Verification items for this drawing (mm, ordinates from the low corner). Give positions to 0.01 mm unless a question says otherwise; leave off trailing zeros. Loops run counter-clockwise (first coordinate to the right, second up) from the corner with the lowest first, then second, coordinate; pieces in that order, holes last. Notation, with made-up numbers: (-16.75, 1) -> (-5.75, 1) arc R27 cw to (-5.75, 30) -> close; hole circle Ø4 at (22.25, -7). An arc over 180 degrees is marked (long way). Answer as a JSON object with one key per item and string values.
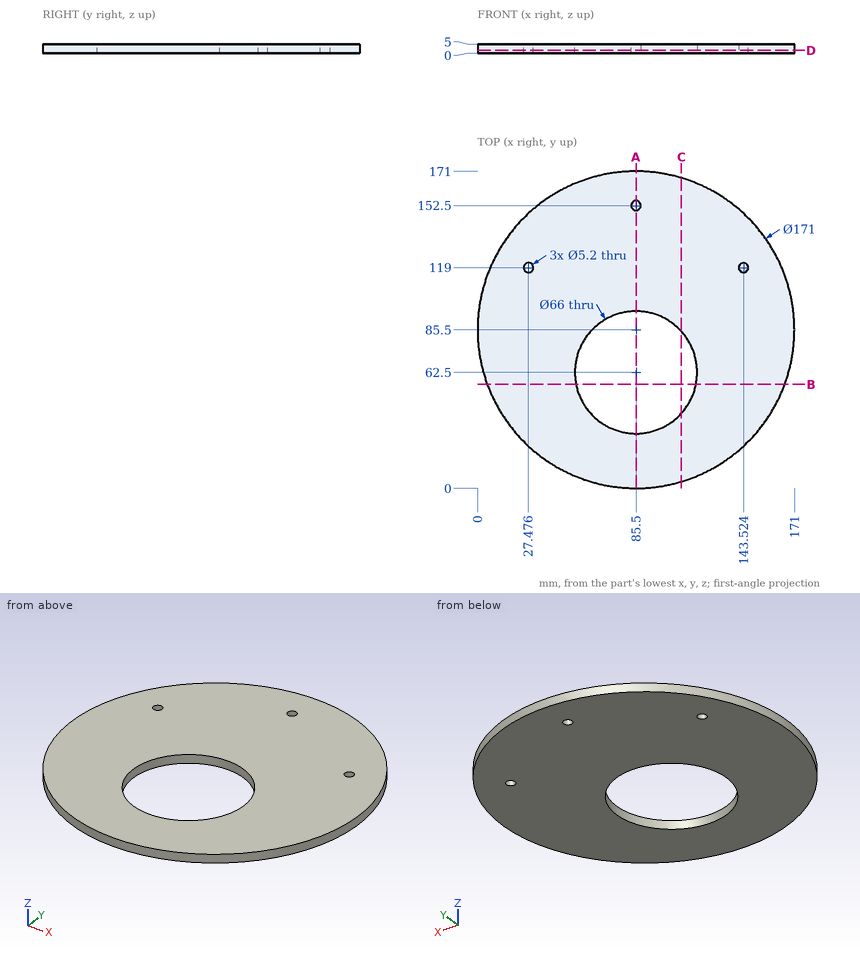
1) Section check B-B on y = 56. Record the cut outline in (x, z), plus the area to 3 significant figures.
Geometry check:
{"outline": "(5.25, 0) -> (53.15, 0) -> (53.15, 5) -> (5.25, 5) -> close; (117.85, 0) -> (165.75, 0) -> (165.75, 5) -> (117.85, 5) -> close", "area": "479 mm2"}
2) Section check C-C on x = 110. Record the cut outline in (y, z) (1 decimal), plus the area to 3 significant figures.
Geometry check:
{"outline": "(3.6, 0) -> (40.4, 0) -> (40.4, 5) -> (3.6, 5) -> close; (84.6, 0) -> (167.4, 0) -> (167.4, 5) -> (84.6, 5) -> close", "area": "598 mm2"}
3) Section check A-A on x = 85.5. Record the cut outline in (y, z).
Geometry check:
{"outline": "(0, 0) -> (29.5, 0) -> (29.5, 5) -> (0, 5) -> close; (95.5, 0) -> (149.9, 0) -> (149.9, 5) -> (95.5, 5) -> close; (155.1, 0) -> (171, 0) -> (171, 5) -> (155.1, 5) -> close"}
4) Material ranges on line 1 along Y through (x, z) = (85.5, 2.3); line 2 along X through (y, z) = (70, 4.3); line 3 along X through (y, z) = (47, 3.1), recorded low to high. Write a range as from..to.
Geometry check:
{"line 1": "y = 0..29.5, 95.5..149.9, 155.1..171", "line 2": "x = 1.42..53.36, 117.64..169.58", "line 3": "x = 9.16..56.37, 114.63..161.84"}
5) Section check D-D on z = 1.55. Record the cut outline in (x, y), plus the area to 3 significant figures.
Geometry check:
{"outline": "circle Ø171 at (85.5, 85.5); hole circle Ø5.2 at (27.48, 119); hole circle Ø66 at (85.5, 62.5); hole circle Ø5.2 at (85.5, 152.5); hole circle Ø5.2 at (143.52, 119)", "area": "19,500 mm2"}
6) Depth check by flat-ended pin: P1, Ø1.5, axis at x = 147, z = 1, coming from the +Y side (1 decimal); P2, Ø4, axis at x = 27.48, y = 119, coming from the -Z side; P3, Ø1.5, axis at y = 53.5, z = 3, coming from the -X side (1 decimal); P4, Ø1, axis at x = 102, z = 3.5, coming from the -Y side. Enter the tip coordinate at first touch or a pass-through.
Geometry check:
{"P1": "stops at y = 145.7", "P2": "passes through", "P3": "stops at x = 5.9", "P4": "stops at y = 1.51"}
